For this review, take the finished solid that the model builds, in its own axes (mm). Face numbers are marked on the shaded views. A direction names the side the tool comes from. Coordinates: 2 decimals unless noted, no trailing zeros. Loops run counter-clockwise (first coordinate to the right, second up) from the corner with the lowest first, then second, coordinate; pieces in that order, holes last.
1. To check wall thickness, follow probe 1 along X at (y, z) = (102, 0); probe 2 along X at (y, z) = (4.25, 0); probe 3 along X at (y, z) = (13, 0). State the ranges of each line that lie inside material, in increasing order.
2. Mouldability with a two-part tool opening along X and no side actions: class the marked faces 4, 5, 6 and 7 as pulls with the +X half, pulls with the -X half, needs draft (parallel to the pull), parting line crosses it, or undercut.
3. Take a section at B-B, the plane y = 84.5. State the section outline as (x, z) points.
4. Take a section at A-A, the plane y = 60.5. State the section outline as (x, z) points, then the cut area to 3 significant figures.
5. Clearance check with flat-ended pins moving along their axes: P1, Ø12, axis at x = -1, z = 23, coming from the -Y side; P2, Ø1.5, axis at y = 54.5, z = -0.5, coming from the -X side; P3, Ø5, axis at x = 29, y = 83.5, coming from the +Z side. State where each tip first meets the part, or that it passes through.
6. Take a section at C-C, the plane x = 0. Count the separate pieces of the cut face and the enclosed holes in it, then the cut area to 3 significant figures.
7. Machinability: for the marked faces 1, 2 and 3, which of the approach directions +Z, -Z, +X, -X, +Y, -Y give a long, thin tool a straight path to every point of the face, cutting with its end or side? Answer none if there is none.
```python
from build123d import *


with BuildPart() as part:
    # Sketch1 → Revolve-Thin2 (revolve)
    with BuildSketch(Plane.XY, mode=Mode.PRIVATE) as revolve_thin2_sk:
        Polygon((-30.568264707, -2), (-39.483227781, -2), (-39.483227781, 7.913824599), (-42.483227781, 7.913824599), (-42.483227781, 92), (-36.483227781, 92), (-36.483227781, 110), (-30.568264707, 110), (-30.568264707, 28.789318309), (-17.568264707, 21.050812692), (-17.568264707, 7.913824599), (-30.568264707, 7.913824599), align=None)
        Polygon((-32.568264707, 0), (-37.483227781, 0), (-37.483227781, 9.913824599), (-40.483227781, 9.913824599), (-40.483227781, 90), (-34.483227781, 90), (-34.483227781, 108), (-32.568264707, 108), (-32.568264707, 27.652330216), (-19.568264707, 19.913824599), (-19.568264707, 9.913824599), (-32.568264707, 9.913824599), align=None, mode=Mode.SUBTRACT)
    revolve(revolve_thin2_sk.sketch.rotate(Axis((0, 0, 0), (0, 1, 0)), 270), axis=Axis((0, 0, 0), (0, 1, 0)))


with BuildPart() as body_2:
    # Sketch2 → Revolve1 (revolve)
    with BuildSketch(Plane.XY, mode=Mode.PRIVATE) as revolve1_sk:
        Polygon((-8, 9.913824599), (-8, 19.5), (-14.206561831, 24.739637185), (-14, 90), (-9.000025046, 89.9841741), (-9.19920546, 27.055868252), (-3, 21.822441383), (-3, 9.913824599), align=None)
    revolve(revolve1_sk.sketch.rotate(Axis((0, 0, 0), (0, 1, 0)), 270), axis=Axis((0, 0, 0), (0, 1, 0)))


with BuildPart() as part_1:
    add(part.part)

    add(body_2.part)  # Revolve4 merges body 2
    # Sketch3 → Revolve4 (revolve)
    with BuildSketch(Plane.XY, mode=Mode.PRIVATE) as revolve4_sk:
        Polygon((-21.027014256, 57.038111316), (-21.027014256, 50.338132018), (-27.983227781, 50.338132018), (-32.562811664, 50.338132018), (-32.562811664, 44.614788696), (0, 44.614788696), (0, 62.838111316), (-27.983227781, 62.838111316), (-32.562811664, 62.838111316), (-32.562811664, 57.038111316), align=None)
    revolve(revolve4_sk.sketch.rotate(Axis((0, 0, 0), (0, 1, 0)), 270), axis=Axis((0, 0, 0), (0, 1, 0)))


solid = part_1.part
```
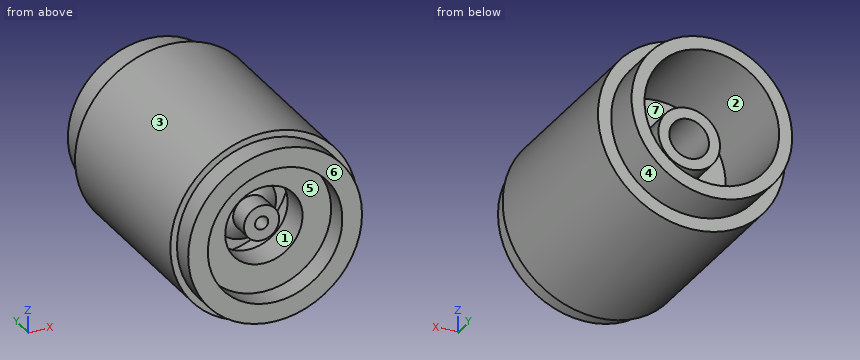
Results list:
1. probe 1: x = -36.48 to -34.48, -32.57 to -30.57, 30.57 to 32.57, 34.48 to 36.48
1. probe 2: x = -39.48 to -37.48, -32.57 to -30.57, 30.57 to 32.57, 37.48 to 39.48
1. probe 3: x = -42.48 to -40.48, -19.57 to -17.57, -8 to -3, 3 to 8, 17.57 to 19.57, 40.48 to 42.48
2. face 4: parting line crosses it
2. face 5: undercut
2. face 6: needs draft
2. face 7: undercut
3. outline: circle Ø84.97 at (0, 0); circle Ø65.14 at (0, 0); circle Ø28.03 at (0, 0); hole circle Ø80.97 at (0, 0); hole circle Ø61.14 at (0, 0); hole circle Ø18.03 at (0, 0)
4. outline: circle Ø84.97 at (0, 0); circle Ø65.14 at (0, 0); hole circle Ø80.97 at (0, 0)
4. area: 3,850 mm2
5. P1: stops at y = 7.91
5. P2: stops at x = -42.48
5. P3: stops at z = 33.21
6. separate pieces: 1
6. enclosed holes: 4
6. area: 2,670 mm2
7. face 1: -Y
7. face 2: +Y
7. face 3: +Y, -Y
